Can you work these out from the model? Positions are in its coordinate system, mm. A direction names the side the tool comes from. Give positions to 0.01 mm unless a question says otherwise; leave off trailing zeros. Write each loop counter-clockwise with the first axis right and the second up, starting at its lowest first coordinate (ties: lowest second). Pieces come first, ordered by that corner, then holes.
1. I'm going to push a flat-ended pin straight in: pin 1 (3 mm diameter, centred on x = -4, y = 35.5, fed in from +Z). Where does the tip first touch, or does it pass through?
2. Suppose I cut it at A-A (z = -7.25). Please give me the cut outline in (x, y), and give its area (3 significant figures).
3. Thinking about a two-plate mould opening in Y: for faces 4 (the flat face through (0, 2, 1.5)), 5 (the flat face through (0, 19, -15)), 6 (the flat face through (0, 38, -10)), 7 (the cylindrical face through (0, 37, 1)), which applies, pulls with the +Y half, pulls with the -Y half, needs draft (parallel to the pull), parting line crosses it, or undercut?
4. Suppose I cut it at B-B (y = 2). Please give me the cut outline in (x, z).
5. If I drill on probe 1 along Y at (x, z) = (-7, -14.75); probe 2 along Z at (x, y) = (-5, 27.5); probe 3 along Z at (x, y) = (9, 3), over which ranges is the centre line in solid material (lowest first)?
6. Suppose I cut it at D-D (x = 0). Please give me the cut outline in (y, z).
7. On a 3-axis mill with a long thin cutter (end or side, diameter ignored), from which of +Z, -Z, +X, -X, +Y, -Y can I reach the whole of each face in a straight line? I mean faces 1 (the flat face through (0, 34, -8)), 2 (the flat face through (16, 19.3, -15.3)), 3 (the cylindrical face through (0, 1, 1)). Say none if no direction works.
8. Suppose I cut it at C-C (x = -3.5). Please give me the cut outline in (y, z).
```python
from build123d import *

# Parameters (mm, degrees)
BOSS_EXTRUDE1_DEPTH = 16
SKETCH4_R           = 1
BOSS_EXTRUDE2_DEPTH = 1.5


with BuildPart() as part:
    # Sketch3 → Boss-Extrude1 (new body, symmetric)
    with BuildSketch(Plane(origin=(0, 0, 0), x_dir=(0, 0, -1), z_dir=(1, 0, 0))):
        Polygon((0, 0), (0, 4), (15, 4), (15, 34), (0, 34), (0, 38), (21, 38), (21, 0), align=None)
    extrude(amount=BOSS_EXTRUDE1_DEPTH, both=True)

    # Sketch4 → Boss-Extrude2 (add, symmetric)
    with BuildSketch(Plane.XY):
        with Locations((0, 36)):
            Circle(SKETCH4_R)
        with Locations((0, 2)):
            Circle(SKETCH4_R)
    extrude(amount=BOSS_EXTRUDE2_DEPTH, both=True)


solid = part.part
```
Checks:
1. pin 1: stops at z = 0
2. outline: (-16, 0) - (16, 0) - (16, 4) - (-16, 4) - close; (-16, 34) - (16, 34) - (16, 38) - (-16, 38) - close
2. area: 256 mm2
3. face 4: needs draft
3. face 5: undercut
3. face 6: pulls with the +Y half
3. face 7: undercut
4. outline: (-16, -21) - (16, -21) - (16, 0) - (1, 0) - (1, 1.5) - (-1, 1.5) - (-1, 0) - (-16, 0) - close
5. probe 1: y = 0 to 4, 34 to 38
5. probe 2: z = -21 to -15
5. probe 3: z = -21 to 0
6. outline: (0, -21) - (38, -21) - (38, 0) - (37, 0) - (37, 1.5) - (35, 1.5) - (35, 0) - (34, 0) - (34, -15) - (4, -15) - (4, 0) - (3, 0) - (3, 1.5) - (1, 1.5) - (1, 0) - (0, 0) - close
7. face 1: +Z, +X, -X
7. face 2: +Z, -Z, +X, +Y, -Y
7. face 3: +Z
8. outline: (0, -21) - (38, -21) - (38, 0) - (34, 0) - (34, -15) - (4, -15) - (4, 0) - (0, 0) - close
